```python
from build123d import *

# Parameters (mm, degrees)
SKETCH1_W           = 56.5
SKETCH1_H           = 56.5
SKETCH1_W_2         = 50.5
SKETCH1_H_2         = 50.5
SKETCH1_R           = 1.65
BOSS_EXTRUDE1_DEPTH = 8.6
SKETCH2_W           = 50.5
SKETCH2_H           = 50.5
SKETCH2_W_2         = 44.5
SKETCH2_H_2         = 44.5
BOSS_EXTRUDE2_DEPTH = 2
BOSS_EXTRUDE3_START = 6.6
SKETCH4_W           = 50.5
SKETCH4_H           = 50.5
SKETCH4_W_2         = 44.5
SKETCH4_H_2         = 44.5
BOSS_EXTRUDE3_DEPTH = 2
CUT_EXTRUDE1_START  = 2
SKETCH5_W           = 6
SKETCH5_H           = 17.961455198
CUT_EXTRUDE1_DEPTH  = 4.6
SKETCH6_W           = 87.3205389
SKETCH6_H           = 82.15723747
CUT_EXTRUDE2_DEPTH  = 2.3


with BuildPart() as part:
    # Sketch1 → Boss-Extrude1 (new body)
    with BuildSketch(Plane(origin=(0, 0, 0), x_dir=(1, 0, 0), z_dir=(0, 1, 0))):
        Rectangle(SKETCH1_W, SKETCH1_H)
        Rectangle(SKETCH1_W_2, SKETCH1_H_2, mode=Mode.SUBTRACT)
        Polygon((-28.25, -28.25), (-28.25, -12.25), (-36.25, -20.25), (-36.25, -30.25), (-32.25, -34.25), (-24.25, -34.25), (-18.25, -28.25), align=None)
        with Locations((-32.25, -24.25)):
            Circle(SKETCH1_R, mode=Mode.SUBTRACT)
        Polygon((28.25, -28.25), (18.25, -28.25), (24.25, -34.25), (32.25, -34.25), (36.25, -30.25), (36.25, -20.25), (28.25, -12.25), align=None)
        with Locations((32.25, -24.25)):
            Circle(SKETCH1_R, mode=Mode.SUBTRACT)
        Polygon((24.25, 34.25), (18.25, 28.25), (28.25, 28.25), (28.25, 12.25), (36.25, 20.25), (36.25, 30.25), (32.25, 34.25), align=None)
        with Locations((32.25, 24.25)):
            Circle(SKETCH1_R, mode=Mode.SUBTRACT)
        Polygon((-36.25, 20.25), (-28.25, 12.25), (-28.25, 28.25), (-18.25, 28.25), (-24.25, 34.25), (-32.25, 34.25), (-36.25, 30.25), align=None)
        with Locations((-32.25, 24.25)):
            Circle(SKETCH1_R, mode=Mode.SUBTRACT)
    extrude(amount=BOSS_EXTRUDE1_DEPTH)

    # Sketch2 → Boss-Extrude2 (add)
    with BuildSketch(Plane(origin=(0, 0, 0), x_dir=(1, 0, 0), z_dir=(0, 1, 0))):
        Rectangle(SKETCH2_W, SKETCH2_H)
        Rectangle(SKETCH2_W_2, SKETCH2_H_2, mode=Mode.SUBTRACT)
    extrude(amount=BOSS_EXTRUDE2_DEPTH)

    # Sketch4 → Boss-Extrude3 (add)
    with BuildSketch(Plane(origin=(0, 0, 0), x_dir=(1, 0, 0), z_dir=(0, 1, 0)).offset(BOSS_EXTRUDE3_START)):
        Rectangle(SKETCH4_W, SKETCH4_H)
        Rectangle(SKETCH4_W_2, SKETCH4_H_2, mode=Mode.SUBTRACT)
    extrude(amount=BOSS_EXTRUDE3_DEPTH)

    # Sketch5 → Cut-Extrude1 (cut)
    with BuildSketch(Plane(origin=(0, 0, 0), x_dir=(1, 0, 0), z_dir=(0, 1, 0)).offset(CUT_EXTRUDE1_START)):
        with Locations((-22.25, 28.869783692)):
            Rectangle(SKETCH5_W, SKETCH5_H)
        with Locations((22.25, 28.869783692)):
            Rectangle(SKETCH5_W, SKETCH5_H)
    extrude(amount=CUT_EXTRUDE1_DEPTH, mode=Mode.SUBTRACT)

    # Sketch6 → Cut-Extrude2 (cut)
    with BuildSketch(Plane.XZ):
        with Locations((1.898272585, -1.518618068)):
            Rectangle(SKETCH6_W, SKETCH6_H)
    extrude(amount=-CUT_EXTRUDE2_DEPTH, mode=Mode.SUBTRACT)


solid = part.part
```
Build history of the part. All positions in model axes, mm. A direction names the side the tool comes from. Round coordinates to 2 decimals unless told otherwise and drop trailing zeros. Write each loop counter-clockwise with the first axis right and the second up, starting at its lowest first coordinate (ties: lowest second). Pieces come first, ordered by that corner, then holes.
1) 3-axis set-ups, long thin cutter, end or side, ignore diameter. For faces 1 (the flat face through (22.25, 8, 0)), 2 (the flat face through (-32, 5, -16)), 3 (the flat face through (25.25, 4, -4)), 4 (the flat face through (0, 5, -28.25)): which of +Z, -Z, +X, -X, +Y, -Y reach the whole face in a straight line?
2) Band-saw the part on C-C, the plane z = 24.25. List the corners of the cut face in (x, y).
3) Pin check, flat tips, straight feed: pin 1 (1 mm diameter, centred on x = 5, y = 7.5, fed in from +Z); pin 2 (1.6 mm diameter, centred on y = 7.5, z = 4.5, fed in from -X); pin 3 (3.5 mm diameter, centred on y = 3.5, z = -11.5, fed in from -X). Stop position of each tip, or through.
4) Drill centre lines: probe 1 along X at (y, z) = (6.25, -24.25); probe 2 along X at (y, z) = (7.25, 4.5); probe 3 along Z at (x, y) = (32.25, 7). Where is each one in solid material? Low to high.
5) Band-saw the part on B-B, the plane z = 16. List the corners of the cut face in (x, y).
6) Band-saw the part on D-D, the plane x = -6. List the corners of the cut face in (y, z).
7) Mould opens along Z. For faces 5 (the cylindrical face through (31.034, 5.406, -25.365)), 6 (the flat face through (28, 5, -34.25)), 7 (the flat face through (0, 5, 28.25)), 8 (the flat face through (0, 4, -25.25)) say: +Z half, -Z half, draft (parallel to the pull), parting line (faces both ways), or undercut.
8) Band-saw the part on A-A, the plane y = 4.25. Give the number of separate pieces and of enclosed holes in the cut face, and give its area (3 significant figures).
Ans:
1. face 1: +Y, -Y
1. face 2: -X, +Y, -Y
1. face 3: -Z, -Y
1. face 4: -Z, +Y, -Y
2. outline: (-36.25, 2.3) - (-33.9, 2.3) - (-33.9, 8.6) - (-36.25, 8.6) - close; (-30.6, 2.3) - (-25.25, 2.3) - (-25.25, 6.6) - (25.25, 6.6) - (25.25, 2.3) - (30.6, 2.3) - (30.6, 8.6) - (-30.6, 8.6) - close; (33.9, 2.3) - (36.25, 2.3) - (36.25, 8.6) - (33.9, 8.6) - close
3. pin 1: stops at z = 28.25
3. pin 2: stops at x = -28.25
3. pin 3: stops at x = -29.25
4. probe 1: x = -36.25 to -33.9, -30.6 to -25.25, 25.25 to 30.6, 33.9 to 36.25
4. probe 2: x = -28.25 to -22.25, 22.25 to 28.25
4. probe 3: z = -34.25 to -25.9, -22.6 to -16.25, 16.25 to 22.6, 25.9 to 34.25
5. outline: (-32, 2.3) - (-25.25, 2.3) - (-25.25, 6.6) - (-22.25, 6.6) - (-22.25, 8.6) - (-32, 8.6) - close; (22.25, 6.6) - (25.25, 6.6) - (25.25, 2.3) - (32, 2.3) - (32, 8.6) - (22.25, 8.6) - close
6. outline: (2.3, -28.25) - (8.6, -28.25) - (8.6, -22.25) - (6.6, -22.25) - (6.6, -25.25) - (2.3, -25.25) - close; (2.3, 25.25) - (6.6, 25.25) - (6.6, 22.25) - (8.6, 22.25) - (8.6, 28.25) - (2.3, 28.25) - close
7. face 5: undercut
7. face 6: -Z half
7. face 7: +Z half
7. face 8: undercut
8. separate pieces: 2
8. enclosed holes: 4
8. area: 1,240 mm2
